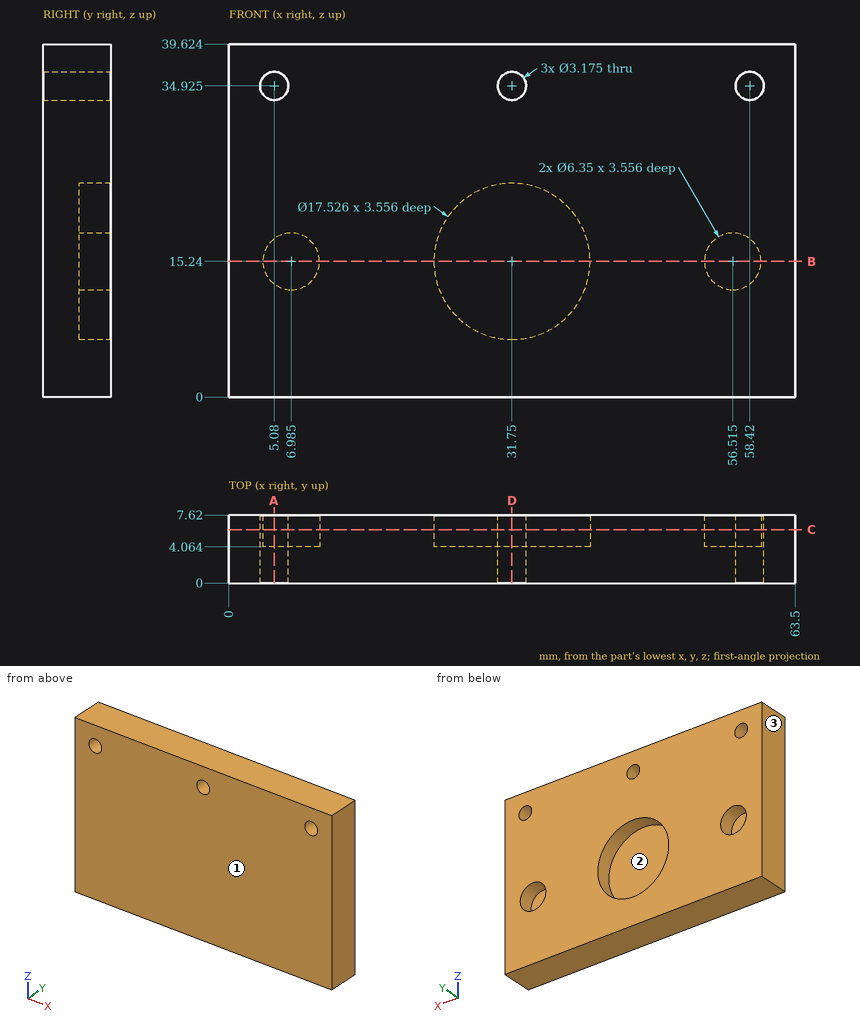
Print and shaded views of the part. All mm, measured from the part's lowest x, y and z. Round coordinates to 2 decimals unless told otherwise and drop trailing zeros. Write each loop counter-clockwise with the first axis right and the second up, starting at its lowest first coordinate (ties: lowest second). Pieces come first, ordered by that corner, then holes. Notation, with made-up numbers: (2, 66) - (23, 66) arc R13 ccw to (23, 82) - close; hole circle Ø9 at (69.5, 40). An arc over 180 degrees is marked (long way). Write each question's results on one line, items separated by ' | '. Start each with the question number.
Item 1: Saw through at C-C (y = 6). State how many separate pieces and enclosed holes the cut face has, and give its area (3 significant figures).
Item 2: Saw through at B-B (z = 15.24). Write the cut outline in (x, y).
Item 3: Saw through at D-D (x = 31.75). Write the cut outline in (y, z), and give its area (3 significant figures).
Item 4: Drop flat-ended pins along their axis: P1, Ø3, axis at x = 7, z = 15, coming from the +Y side; P2, Ø2.5, axis at x = 5.08, z = 34.925, coming from the -Y side. Give the stop position or say it passes through.
Item 5: Saw through at A-A (x = 5.08). Write the cut outline in (y, z), and give its area (3 significant figures).
Item 6: Mould opens along X. For the marked faces 1, 2 and 3 say: pulls with the +X half, pulls with the -X half, needs draft (parallel to the pull), parting line crosses it, or undercut.
Item 7: Wall check: L1, parallel to X at y = 5.45, z = 15.24; L2, parallel to X at y = 6, z = 36; L3, parallel to Y at x = 26.5, z = 17. Give the ranges that are in metal, low to high. Write a range as [from, to].
Results are:
1) separate pieces: 1 | enclosed holes: 6 | area: 2,190 mm²
2) outline: (0, 0) - (63.5, 0) - (63.5, 7.62) - (59.69, 7.62) - (59.69, 4.06) - (53.34, 4.06) - (53.34, 7.62) - (40.51, 7.62) - (40.51, 4.06) - (22.99, 4.06) - (22.99, 7.62) - (10.16, 7.62) - (10.16, 4.06) - (3.81, 4.06) - (3.81, 7.62) - (0, 7.62) - close
3) outline: (0, 0) - (7.62, 0) - (7.62, 6.48) - (4.06, 6.48) - (4.06, 24) - (7.62, 24) - (7.62, 33.34) - (0, 33.34) - close; (0, 36.51) - (7.62, 36.51) - (7.62, 39.62) - (0, 39.62) - close | area: 215 mm²
4) P1: stops at y = 4.06 | P2: passes through
5) outline: (0, 0) - (7.62, 0) - (7.62, 12.7) - (4.06, 12.7) - (4.06, 17.78) - (7.62, 17.78) - (7.62, 33.34) - (0, 33.34) - close; (0, 36.51) - (7.62, 36.51) - (7.62, 39.62) - (0, 39.62) - close | area: 260 mm²
6) face 1: needs draft | face 2: undercut | face 3: pulls with the -X half
7) L1: x = [0, 3.81], [10.16, 22.99], [40.51, 53.34], [59.69, 63.5] | L2: x = [0, 3.91], [6.25, 30.58], [32.92, 57.25], [59.59, 63.5] | L3: y = [0, 4.06]
